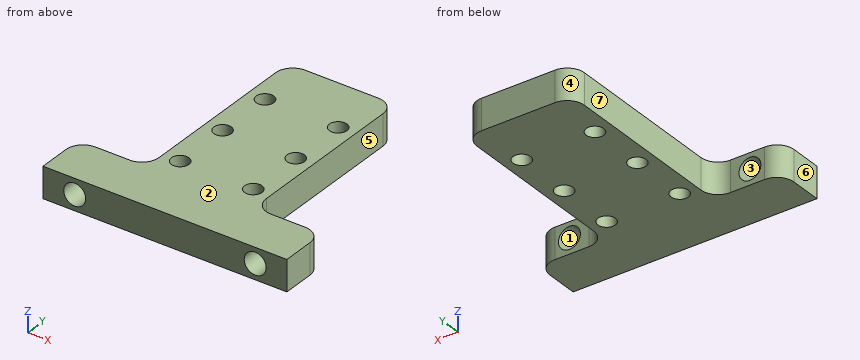
```python
from build123d import *

# Parameters (mm, degrees)
BOSS_EXTRUDE1_DEPTH  = 6.35
M4_CLEARANCE_HOLE1_D = 4.5
M3_CLEARANCE_HOLE2_D = 3.6
FILLET1_R            = 3.5
FILLET2_R            = 3.5


with BuildPart() as part:
    # Sketch1 → Boss-Extrude1 (new body)
    with BuildSketch(Plane.XY):
        Polygon((-25, 0), (25, 0), (25, 10), (11, 10), (11, 50), (-11, 50), (-11, 10), (-25, 10), align=None)
    extrude(amount=BOSS_EXTRUDE1_DEPTH)

    # M4 Clearance Hole1 (through all)
    with Locations(Plane(origin=(0, 10, 0), x_dir=(1, 0, 0), z_dir=(0, 1, 0))):
        with Locations((-18.5, -3.175), (18.5, -3.175)):
            Hole(M4_CLEARANCE_HOLE1_D / 2)

    # M3 Clearance Hole2 (through all)
    with Locations(Plane.XY.offset(6.35)):
        with Locations((-7.5, 26.65), (7.5, 38.65), (-7.5, 14.65), (7.5, 26.65), (-7.5, 38.65), (7.5, 14.65)):
            Hole(M3_CLEARANCE_HOLE2_D / 2)

    # Fillet1
    fillet1_edges = [part.edges().sort_by_distance(p)[0] for p in [
        (-11, 10, 3.175),
        (11, 10, 3.175),
    ]]
    fillet(fillet1_edges, radius=FILLET1_R)

    # Fillet2
    fillet2_edges = [part.edges().sort_by_distance(p)[0] for p in [
        (-25, 10, 3.175),
        (-11, 50, 3.175),
        (11, 50, 3.175),
        (25, 10, 3.175),
    ]]
    fillet(fillet2_edges, radius=FILLET2_R)


solid = part.part
```
Work out the finished part from the listing and answer in its coordinate system (mm). Face numbers are marked on the shaded views. A direction names the side the tool comes from. Give positions to 0.01 mm unless a question says otherwise; leave off trailing zeros. Order: outer loops, then holes, each group sorted by start corner. A loop starts at its lowest first (then second) coordinate and runs counter-clockwise, first axis right, second up. Notation, with made-up numbers: M -8.5,80.5 L 13.5,80.5 A16 ccw 13.5,96.5 Z; hole C 12,24 d7. An arc over 180 degrees is marked long. Return JSON: item names as keys, results as strings.
1) Section C-C, the plane y = 26.65 is taken. Write down the section's boundary in (x, z).
Resolved:
{"outline": "M -11,0 L -9.3,0 L -9.3,6.35 L -11,6.35 Z; M -5.7,0 L 5.7,0 L 5.7,6.35 L -5.7,6.35 Z; M 9.3,0 L 11,0 L 11,6.35 L 9.3,6.35 Z"}
2) Section A-A, the plane x = -18.5 is taken. Write down the section's boundary in (y, z) (3 decimals), plus the area to 3 significant figures.
Resolved:
{"outline": "M 0,0 L 10,0 L 10,0.925 L 0,0.925 Z; M 0,5.425 L 10,5.425 L 10,6.35 L 0,6.35 Z", "area": "18.5 mm^2"}
3) Each of these flat-tipped pins is pushed along its axis until it touches: pin 1 (3 mm diameter, centred on x = -7.5, y = 14.65, fed in from -Z); pin 2 (1.5 mm diameter, centred on y = 33, z = 1, fed in from +X); pin 3 (1 mm diameter, centred on x = -16, z = 5, fed in from +Y). Where does it stop, or does it pass through?
Resolved:
{"pin 1": "through", "pin 2": "x = 11", "pin 3": "y = 10"}
4) A tool of negligible diameter and unlimited length cuts with its end or side. For the marked faces 5, 6 and 7, from which of +Z, -Z, +X, -X, +Y, -Y can it reach the whole face along a straight path? Write none if from no direction.
Resolved:
{"face 5": "+Z, -Z, +X, +Y", "face 6": "+Z, -Z, -X, +Y, -Y", "face 7": "+Z, -Z, -X, +Y"}
5) Section B-B, the plane z = 4.5 is taken. Give the number of separate pieces and of enclosed holes in the cut face, plus the area to 3 significant figures.
Resolved:
{"separate pieces": "3", "enclosed holes": "6", "area": "1,240 mm^2"}
6) For a pull along X with two mould halves and no side action, classify the marked faces 1, 2, 3 and 4 as +X half, -X half, draft (parallel to the pull), parting line (faces both ways), or undercut.
Resolved:
{"face 1": "undercut", "face 2": "draft", "face 3": "undercut", "face 4": "-X half"}
7) Straight lines are drawn through the part: line 1 along Y through (x, z) = (7.5, 2.5); line 2 along X through (y, z) = (38, 2.25); line 3 along X through (y, z) = (13.5, 4.75). For each, find the intervals that lie inside material, in ascending order. Write a range as [from, to].
Resolved:
{"line 1": "[0, 12.85], [16.45, 24.85], [28.45, 36.85], [40.45, 50]", "line 2": "[-11, -9.18], [-5.82, 5.82], [9.18, 11]", "line 3": "[-11, -8.88], [-6.12, 6.12], [8.88, 11]"}
